Work out the finished part from the listing and answer in its coordinate system (mm). A direction names the side the tool comes from. Round coordinates to 2 decimals unless told otherwise and drop trailing zeros. Write each loop counter-clockwise with the first axis right and the second up, starting at its lowest first coordinate (ties: lowest second). Pieces come first, ordered by that corner, then holes. Notation, with made-up numbers: (43.25, 41.5) -> (100.25, 41.5) arc R31 ccw to (100.25, 72.5) -> close; hole circle Ø6 at (-29.75, 23.25). An arc over 180 degrees is marked (long way). One line per item, written item: value.
```python
from build123d import *

# Parameters (mm, degrees)
SKETCH1_R                    = 20
PCB_DEPTH                    = 1
SKETCH2_W                    = 18
SKETCH2_H                    = 4
HIROSE_CONNECTOR_STACK_DEPTH = 2
CIRPATTERN1_COUNT            = 4


with BuildPart() as part:
    # Sketch1 → PCB (new body)
    with BuildSketch(Plane(origin=(0, 0, 0), x_dir=(1, 0, 0), z_dir=(0, 1, 0))):
        with Locations(Location((0, 0, 0), (0, 0, 270))):
            Circle(SKETCH1_R)
    extrude(amount=PCB_DEPTH)

    # Sketch2 → Hirose Connector Stack (add)
    with BuildSketch(Plane(origin=(0, 1, 0), x_dir=(1, 0, 0), z_dir=(0, 1, 0))):
        with Locations((0, 14)):
            Rectangle(SKETCH2_W, SKETCH2_H)
    hirose_connector_stack = extrude(amount=HIROSE_CONNECTOR_STACK_DEPTH)

    # CirPattern1: Hirose Connector Stack ×4 about axis
    cirpattern1_axis = Axis((0, 0, 0), (0, 1, 0))
    for i in range(1, CIRPATTERN1_COUNT):
        add(hirose_connector_stack.rotate(cirpattern1_axis, i * 360 / CIRPATTERN1_COUNT))


solid = part.part
```
(1) Flat-ended cylindrical pins translate along their axes: pin 1 Ø0.6 at (y, z) = (2.5, -13.5) entering from +X; pin 2 Ø1.5 at (y, z) = (1.5, -9) entering from +X; pin 3 Ø0.6 at (x, y) = (13.5, 2) entering from +Z. Find the tip coordinate at first contact, or state that the pin passes through.
Reported:
pin 1: stops at x = 9
pin 2: stops at x = 18.13
pin 3: stops at z = 9
(2) Find section A-A on y = 2.55. Give the vertices of the cut face in (x, z), plus the area to 3 significant figures.
Reported:
outline: (-16, -9) -> (-12, -9) -> (-12, 9) -> (-16, 9) -> close; (-9, -16) -> (9, -16) -> (9, -12) -> (-9, -12) -> close; (-9, 12) -> (9, 12) -> (9, 16) -> (-9, 16) -> close; (12, -9) -> (16, -9) -> (16, 9) -> (12, 9) -> close
area: 288 mm2
(3) For a pull along X with two mould halves and no side action, classify faces 1 (the face through (0, 0, 0)), 2 (the face through (12, 2, 0)), 3 (the face through (9, 2, -14)) as pulls with the +X half, pulls with the -X half, needs draft (parallel to the pull), parting line crosses it, or undercut.
Reported:
face 1: needs draft
face 2: undercut
face 3: pulls with the +X half
(4) Find section D-D on y = 0.45. Give the vertices of the cut face in (x, z).
Reported:
outline: circle Ø40 at (0, 0)
(5) A tool of negligible diameter and unlimited length cuts with its end or side. For faces 4 (the face through (14, 2, 9)), 5 (the face through (16, 2, 0)), 6 (the face through (-9, 2, 14)), from which of +Z, -Z, +X, -X, +Y, -Y can it reach the whole face along a straight path? Write none if from no direction.
Reported:
face 4: +Z, +X, -X, +Y
face 5: +Z, -Z, +X, +Y
face 6: +Z, -Z, -X, +Y
(6) Find section C-C on x = -4. Give the vertices of the cut face in (y, z), plus the area to 3 significant figures.
Reported:
outline: (0, -19.6) -> (1, -19.6) -> (1, -16) -> (3, -16) -> (3, -12) -> (1, -12) -> (1, 12) -> (3, 12) -> (3, 16) -> (1, 16) -> (1, 19.6) -> (0, 19.6) -> close
area: 55.2 mm2
(7) Consider probe 1 along Z at (x, y) = (-6, 2.75); probe 2 along Y at (x, z) = (-3.5, 8); probe 3 along X at (y, z) = (1.75, -15.5). Determine where each line is inside the solid, lowest interval first.
Reported:
probe 1: z = -16 to -12, 12 to 16
probe 2: y = 0 to 1
probe 3: x = -9 to 9
(8) Find section B-B on z = 0. Give the vertices of the cut face in (x, y), plus the area to 3 significant figures.
Reported:
outline: (-20, 0) -> (20, 0) -> (20, 1) -> (16, 1) -> (16, 3) -> (12, 3) -> (12, 1) -> (-12, 1) -> (-12, 3) -> (-16, 3) -> (-16, 1) -> (-20, 1) -> close
area: 56.0 mm2
